from build123d import *

# Parameters (mm, degrees)
F0_W     = 63.5
F0_H     = 63.5
F0_W_2   = 1219.2
F1_DEPTH = 6.35
F0_H_2   = 609.6
F2_DEPTH = 6.35


with BuildPart() as f1:
    # F0 (on Top) → F1 (new body)
    with BuildSketch(Plane.XY):
        with Locations((-1312.078089, 1241.172938)):
            Rectangle(F0_W, F0_H)
        with Locations((-1312.078089, 568.072938)):
            Rectangle(F0_W, F0_H)
        with Locations((-670.728089, 1241.172938)):
            Rectangle(F0_W_2, F0_H)
        with Locations((-670.728089, 568.072938)):
            Rectangle(F0_W_2, F0_H)
        Polygon((-61.128089, 1272.922938), (-61.128089, 1209.422938), (-61.128089, 599.822938), (-61.128089, 536.322938), (2.371911, 536.322938), (2.371911, 1272.922938), align=None)
    extrude(amount=F1_DEPTH)

    # F0 (on Top) → F2 (join)
    with BuildSketch(Plane.XY):
        with Locations((-1312.078089, 904.622938)):
            Rectangle(F0_W, F0_H_2)
    extrude(amount=F2_DEPTH)


solid = f1.part
The model under review builds one solid part; all positions refer to its coordinate system, in mm. Coordinates: 2 decimals unless noted, no trailing zeros. Loops run counter-clockwise (first coordinate to the right, second up) from the corner with the lowest first, then second, coordinate; pieces in that order, holes last.
(1) Consider section A-A, the plane x = -531.5. Give the boundary of the cut face in (y, z).
Determined:
outline: (536.32, 0) - (599.82, 0) - (599.82, 6.35) - (536.32, 6.35) - close; (1209.42, 0) - (1272.92, 0) - (1272.92, 6.35) - (1209.42, 6.35) - close
(2) Wall thickness on L1, parallel to X at y = 764.5, z = 0.5; L2, parallel to Y at x = -1280, z = 5: over which ranges is each line inside the solid? List them lowest first.
Determined:
L1: x = -1343.83 to -1280.33, -61.13 to 2.37
L2: y = 536.32 to 599.82, 1209.42 to 1272.92
(3) Consider section C-C, the plane z = 5. Give the boundary of the cut face in (x, y), plus the area to 3 significant figures.
Determined:
outline: (-1343.83, 536.32) - (2.37, 536.32) - (2.37, 1272.92) - (-1343.83, 1272.92) - close; hole (-1280.33, 599.82) - (-61.13, 599.82) - (-61.13, 1209.42) - (-1280.33, 1209.42) - close
area: 248,000 mm2
(4) Draft analysis for pull direction Z (two halves, no side actions). For faces 1 (the flat face through (-724, 579, 0)), 2 (the flat face through (-724, 579, 6.35)), state which applies: +Z half, -Z half, draft (parallel to the pull), parting line (faces both ways), or undercut.
Determined:
face 1: -Z half
face 2: +Z half
(5) Consider section B-B, the plane y = 736. Give the boundary of the cut face in (x, z), plus the area to 3 significant figures.
Determined:
outline: (-1343.83, 0) - (-1280.33, 0) - (-1280.33, 6.35) - (-1343.83, 6.35) - close; (-61.13, 0) - (2.37, 0) - (2.37, 6.35) - (-61.13, 6.35) - close
area: 806 mm2
